The figure shows three views and two pictorial views of one solid part (mm, origin at its lowest corner). Answer the questions. A direction names the side the tool comes from. Round coordinates to 2 decimals unless told otherwise and drop trailing zeros. Loops run counter-clockwise (first coordinate to the right, second up) from the corner with the lowest first, then second, coordinate; pieces in that order, holes last. Notation, with made-up numbers: (32.25, 80) -> (47.25, 80) arc R19 ccw to (47.25, 107) -> close; hole circle Ø3 at (21.5, 22.25). An arc over 180 degrees is marked (long way). Put each result on its own line as item: value.
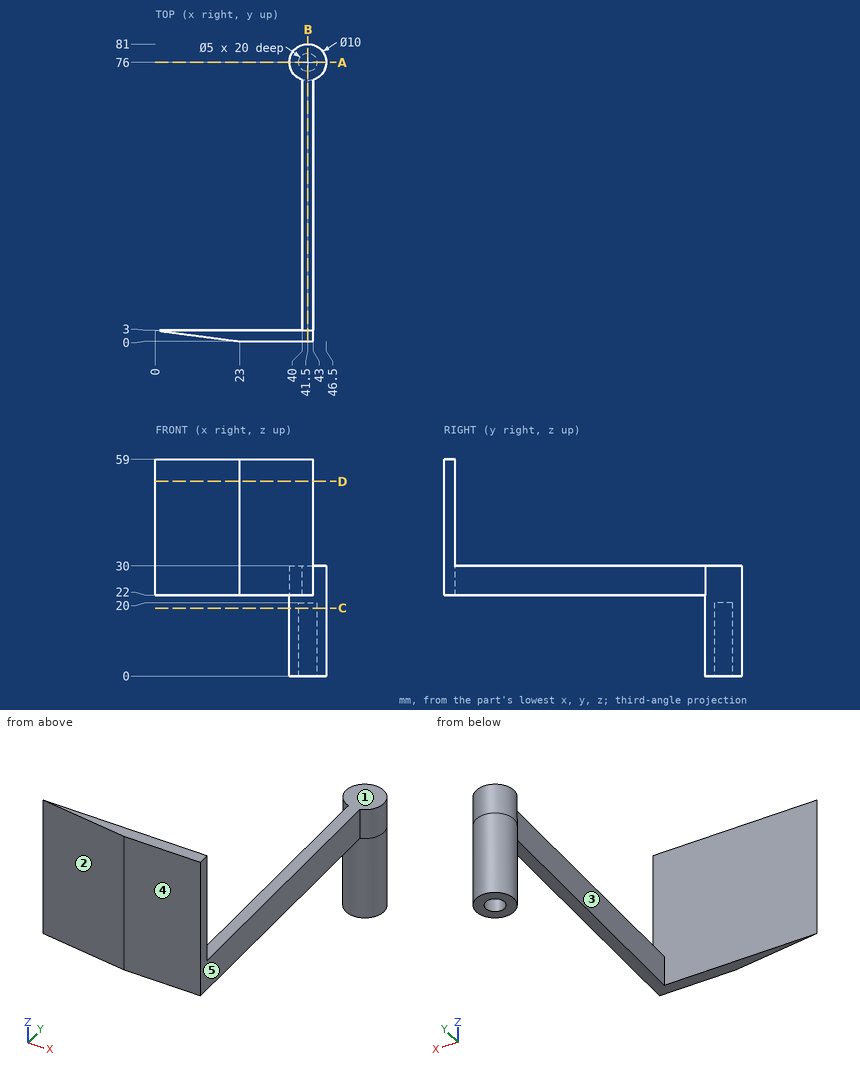
Item 1: Which of the six approach directions +Z, -Z, +X, -X, +Y, -Y give full straight-line access (tool end or side, diameter ignored) to the marked faces 4 and 5?
Derived:
face 4: +Z, -Z, +X, -X, -Y
face 5: +Z, -Z, +X, -Y
Item 2: The part is cut by section D-D (z = 53). Determine the outline of the cut face in (x, y).
Derived:
outline: (0, 3) -> (23, 0) -> (43, 0) -> (43, 3) -> close
Item 3: Flat-ended cylindrical pins translate along their axes: pin 1 Ø4.5 at (x, y) = (41.5, 76) entering from +Z; pin 2 Ø4 at (x, z) = (22, 43) entering from +Y; pin 3 Ø6.5 at (y, z) = (41.5, 26.5) entering from -X. Find the tip coordinate at first contact, or state that the pin passes through.
Derived:
pin 1: stops at z = 30
pin 2: stops at y = 3
pin 3: stops at x = 40
Item 4: The part is cut by section C-C (z = 18.5). Determine the outline of the cut face in (x, y).
Derived:
outline: circle Ø10 at (41.5, 76); hole circle Ø5 at (41.5, 76)
Item 5: For a pull along Y with two mould halves and no side action, classify the marked faces 1, 2 and 3 as pulls with the +Y half, pulls with the -Y half, needs draft (parallel to the pull), parting line crosses it, or undercut.
Derived:
face 1: needs draft
face 2: pulls with the -Y half
face 3: undercut
Item 6: The part is cut by section A-A (y = 76). Determine the outline of the cut face in (x, z), then the cut area to 3 significant figures.
Derived:
outline: (36.5, 0) -> (39, 0) -> (39, 20) -> (44, 20) -> (44, 0) -> (46.5, 0) -> (46.5, 30) -> (36.5, 30) -> close
area: 200 mm^2
Item 7: The part is cut by section B-B (x = 41.5). Determine the outline of the cut face in (y, z), then the cut area to 3 significant figures.
Derived:
outline: (0, 22) -> (71, 22) -> (71, 0) -> (73.5, 0) -> (73.5, 20) -> (78.5, 20) -> (78.5, 0) -> (81, 0) -> (81, 30) -> (3, 30) -> (3, 59) -> (0, 59) -> close
area: 855 mm^2
Item 8: Find the intervals of material crossed by line 1 along Y through (x, z) = (41.5, 10.5); line 2 along Z through (x, y) = (41.5, 20); line 3 along Y through (x, z) = (43, 6.5), in increasing order.
Derived:
line 1: y = 71 to 73.5, 78.5 to 81
line 2: z = 22 to 30
line 3: y = 71.23 to 74, 78 to 80.77
